from build123d import *

# Parameters (mm, degrees)
SKETCH1_W                   = 50
SKETCH1_H                   = 36
BOSS_EXTRUDE1_DEPTH         = 4
SKETCH2_W                   = 30
SKETCH2_H                   = 3
BOSS_EXTRUDE2_DEPTH         = 37
SKETCH3_R                   = 1.55
CUT_EXTRUDE1_DEPTH          = 72.867934435
SKETCH4_W                   = 16
SKETCH4_H                   = 11
CUT_EXTRUDE2_DEPTH          = 10
CUT_EXTRUDE3_DEPTH          = 10
SKETCH6_W                   = 20
SKETCH6_H                   = 12
CUT_EXTRUDE4_DEPTH          = 8
SKETCH7_W                   = 30
SKETCH7_H                   = 3
BOSS_EXTRUDE3_DEPTH         = 2
CHAMFER1_SIZE               = 2
CIRPATTERN1_COUNT           = 2
CIRPATTERN1_COPY_1_DEPTH    = 10
SKETCH9_W                   = 5
SKETCH9_H                   = 36
CUT_EXTRUDE6_DEPTH          = 10
CHAMFER2_SIZE               = 0.5
SKETCH10_W                  = 30
SKETCH10_H                  = 2
BOSS_EXTRUDE4_DEPTH         = 2
CHAMFER3_SIZE               = 2
CUT_EXTRUDE7_START          = -1.5
SKETCH12_W                  = 12.2
SKETCH12_H                  = 5.7
CUT_EXTRUDE7_DEPTH          = 7.5
CIRPATTERN2_COUNT           = 2
CIRPATTERN2_START           = -1.5
CIRPATTERN2_COPY_1_SKETCH_W = 12.2
CIRPATTERN2_COPY_1_SKETCH_H = 5.7
CIRPATTERN2_COPY_1_DEPTH    = 7.5
CHAMFER4_SIZE               = 2


with BuildPart() as part:
    # Sketch1 → Boss-Extrude1 (new body)
    with BuildSketch(Plane.XY):
        with Locations((25, 18)):
            Rectangle(SKETCH1_W, SKETCH1_H)
    extrude(amount=BOSS_EXTRUDE1_DEPTH)

    # Sketch2 → Boss-Extrude2 (add)
    with BuildSketch(Plane(origin=(0, 0, 0), x_dir=(-1, 0, 0), z_dir=(0, 0, -1))):
        with Locations((-35, 34.5)):
            Rectangle(SKETCH2_W, SKETCH2_H)
        with Locations((-35, 1.5)):
            Rectangle(SKETCH2_W, SKETCH2_H)
    extrude(amount=-BOSS_EXTRUDE2_DEPTH)

    # Sketch3 → Cut-Extrude1 (cut, through all)
    with BuildSketch(Plane(origin=(0, 36, 0), x_dir=(1, 0, 0), z_dir=(0, 1, 0))):
        with Locations(Location((40, -30, 0), (0, 0, 270))):
            Circle(SKETCH3_R)
    extrude(amount=-CUT_EXTRUDE1_DEPTH, mode=Mode.SUBTRACT)

    # Sketch4 → Cut-Extrude2 (cut)
    with BuildSketch(Plane(origin=(0, 0, 0), x_dir=(-1, 0, 0), z_dir=(0, 0, -1))):
        with Locations((-27, 18)):
            Rectangle(SKETCH4_W, SKETCH4_H)
    extrude(amount=-CUT_EXTRUDE2_DEPTH, mode=Mode.SUBTRACT)

    # Sketch5 → Cut-Extrude3 (cut)
    with BuildSketch(Plane(origin=(0, 0, 0), x_dir=(-1, 0, 0), z_dir=(0, 0, -1))):
        with BuildLine():
            Line((-44, 14.25), (-38, 14.25))
            ThreePointArc((-38, 14.25), (-36.25, 12.5), (-38, 10.75))
            Line((-38, 10.75), (-44, 10.75))
            ThreePointArc((-44, 10.75), (-45.75, 12.5), (-44, 14.25))
        make_face()
    cut_extrude3 = extrude(amount=-CUT_EXTRUDE3_DEPTH, mode=Mode.SUBTRACT)

    # Mirror1: Cut-Extrude3 across plane
    add(cut_extrude3.mirror(Plane.ZX.offset(22)), mode=Mode.SUBTRACT)

    # Sketch6 → Cut-Extrude4 (cut)
    with BuildSketch(Plane(origin=(0, 0, 0), x_dir=(-1, 0, 0), z_dir=(0, 0, -1))):
        with Locations((-52.25, 22)):
            Rectangle(SKETCH6_W, SKETCH6_H)
    cut_extrude4 = extrude(amount=-CUT_EXTRUDE4_DEPTH, mode=Mode.SUBTRACT)

    # Sketch7 → Boss-Extrude3 (add)
    with BuildSketch(Plane(origin=(0, 3, 0), x_dir=(1, 0, 0), z_dir=(0, 1, 0))):
        with Locations((35, -23.2)):
            Rectangle(SKETCH7_W, SKETCH7_H)
    boss_extrude3 = extrude(amount=BOSS_EXTRUDE3_DEPTH)

    # Mirror3: Boss-Extrude3 across plane
    add(boss_extrude3.mirror(Plane.ZX.offset(18)))

    # Chamfer1
    chamfer1_edges = [part.edges().sort_by_distance(p)[0] for p in [
        (35, 33, 21.7),
        (35, 3, 21.7),
    ]]
    chamfer(chamfer1_edges, length=CHAMFER1_SIZE - 0.0001)  # a hair under: the kernel refuses the full size

    # CirPattern1: Cut-Extrude3, Cut-Extrude4 ×2 about axis
    cirpattern1_axis = Axis((27, 18, 0), (0, 0, 1))
    add([cut_extrude3.rotate(cirpattern1_axis, i * 360 / CIRPATTERN1_COUNT) for i in range(1, CIRPATTERN1_COUNT)], mode=Mode.SUBTRACT)
    add([cut_extrude4.rotate(cirpattern1_axis, i * 360 / CIRPATTERN1_COUNT) for i in range(1, CIRPATTERN1_COUNT)], mode=Mode.SUBTRACT)

    # CirPattern1 copy 1 sketch → CirPattern1 copy 1 (cut)
    with BuildSketch(Plane(origin=(54, -8, 0), x_dir=(1, 0, 0), z_dir=(0, 0, -1))):
        with BuildLine():
            Line((-44, -14.25), (-38, -14.25))
            ThreePointArc((-38, -14.25), (-36.25, -12.5), (-38, -10.75))
            Line((-38, -10.75), (-44, -10.75))
            ThreePointArc((-44, -10.75), (-45.75, -12.5), (-44, -14.25))
        make_face()
    extrude(amount=-CIRPATTERN1_COPY_1_DEPTH, mode=Mode.SUBTRACT)

    # Sketch9 → Cut-Extrude6 (cut)
    with BuildSketch(Plane(origin=(0, 0, 0), x_dir=(-1, 0, 0), z_dir=(0, 0, -1))):
        with Locations((-2.5, 18)):
            Rectangle(SKETCH9_W, SKETCH9_H)
    extrude(amount=-CUT_EXTRUDE6_DEPTH, mode=Mode.SUBTRACT)

    # Chamfer2
    chamfer2_edges = [part.edges().sort_by_distance(p)[0] for p in [
        (41, 29.75, 0),
        (45.75, 31.5, 0),
        (36.25, 31.5, 0),
        (41, 33.25, 0),
        (50, 32, 0),
        (46.125, 28, 0),
        (46.125, 16, 0),
        (42.25, 22, 0),
        (8.25, 23.5, 0),
        (13, 25.25, 0),
        (17.75, 23.5, 0),
        (13, 21.75, 0),
        (8.25, 4.5, 0),
        (13, 2.75, 0),
        (17.75, 4.5, 0),
        (13, 6.25, 0),
        (8.375, 8, 0),
        (11.75, 14, 0),
        (8.375, 20, 0),
        (27.5, 0, 0),
        (5, 28, 0),
        (5, 4, 0),
        (27.5, 36, 0),
        (50, 8, 0),
        (35, 18, 0),
        (27, 12.5, 0),
        (19, 18, 0),
        (27, 23.5, 0),
        (45.75, 12.5, 0),
        (41, 10.75, 0),
        (36.25, 12.5, 0),
        (41, 14.25, 0),
    ]]
    chamfer(chamfer2_edges, length=CHAMFER2_SIZE)

    # Sketch10 → Boss-Extrude4 (add)
    with BuildSketch(Plane(origin=(0, 3, 0), x_dir=(1, 0, 0), z_dir=(0, 1, 0))):
        with Locations((35, -36)):
            Rectangle(SKETCH10_W, SKETCH10_H)
    boss_extrude4 = extrude(amount=BOSS_EXTRUDE4_DEPTH)

    # Mirror4: Boss-Extrude4 across plane
    add(boss_extrude4.mirror(Plane.ZX.offset(18)))

    # Chamfer3
    chamfer3_edges = [part.edges().sort_by_distance(p)[0] for p in [
        (35, 31, 37),
        (35, 5, 37),
    ]]
    chamfer(chamfer3_edges, length=CHAMFER3_SIZE - 0.0001)  # a hair under: the kernel refuses the full size

    # Sketch12 → Cut-Extrude7 (cut)
    with BuildSketch(Plane.XY.offset(4).offset(CUT_EXTRUDE7_START)):
        with Locations((13, 23.5)):
            Rectangle(SKETCH12_W, SKETCH12_H)
    cut_extrude7 = extrude(amount=CUT_EXTRUDE7_DEPTH, mode=Mode.SUBTRACT)

    # Mirror5: Cut-Extrude7 across plane
    add(cut_extrude7.mirror(Plane(origin=(0, 14, 0), x_dir=(0, 0, 1), z_dir=(0, -1, 0))), mode=Mode.SUBTRACT)

    # CirPattern2: Cut-Extrude7 ×2 about axis
    cirpattern2_axis = Axis((27, 18, 0), (0, 0, 1))
    for i in range(1, CIRPATTERN2_COUNT):
        add(cut_extrude7.rotate(cirpattern2_axis, i * 360 / CIRPATTERN2_COUNT), mode=Mode.SUBTRACT)

    # CirPattern2 copy 1 sketch → CirPattern2 copy 1 (cut)
    with BuildSketch(Plane(origin=(54, 8, 4), x_dir=(-1, 0, 0), z_dir=(0, 0, 1)).offset(CIRPATTERN2_START)):
        with Locations((13, -23.5)):
            Rectangle(CIRPATTERN2_COPY_1_SKETCH_W, CIRPATTERN2_COPY_1_SKETCH_H)
    extrude(amount=CIRPATTERN2_COPY_1_DEPTH, mode=Mode.SUBTRACT)

    # Chamfer4
    chamfer4_edges = [part.edges().sort_by_distance(p)[0] for p in [
        (48.55, 33, 4),
        (35, 3, 4),
        (27.45, 33, 4),
    ]]
    chamfer(chamfer4_edges, length=CHAMFER4_SIZE)


solid = part.part
Here's how the part is built. I have some questions about the finished solid (model axes, mm). A direction names the side the tool comes from. Round coordinates to 2 decimals unless told otherwise and drop trailing zeros. Loops run counter-clockwise (first coordinate to the right, second up) from the corner with the lowest first, then second, coordinate; pieces in that order, holes last.
1. We'd pull the mould along X, two halves only. Please class faces 1 (the face through (19, 18, 2)), 2 (the face through (27, 26, 0)), 3 (the face through (20, 2, 21)): +X half, -X half, draft (parallel to the pull), parting line (faces both ways), or undercut.
Answer list:
face 1: undercut
face 2: draft
face 3: -X half
2. For P1, Ø1.5, axis at x = 33, y = 13, coming from the +Z side; P2, Ø1, axis at x = 29.5, y = 4, coming from the +Z side, each with a flat end and sliding along its axis, tell me the tip position at first contact or that it passes through.
Answer list:
P1: stops at z = 4
P2: stops at z = 36.5
3. If I drill on line 1 along X through (y, z) = (34, 30); line 2 along Y through (x, z) = (42.5, 17); line 3 along Y through (x, z) = (28, 24), over which ranges is the centre line in solid material (lowest first)?
Answer list:
line 1: x = 20 to 38.45, 41.55 to 50
line 2: y = 0 to 3, 33 to 36
line 3: y = 0 to 5, 31 to 36
4. If we section it at D-D on x = 40: Count the separate pieces of the cut face and the enclosed holes in it, plus the area to 3 significant figures.
Answer list:
separate pieces: 5
enclosed holes: 0
area: 302 mm2
5. Which directions (+Z, -Z, +X, -X, +Y, -Y) give clear straight access to the entire face, cutting with the end or side of a thin tool? Please do faces 4 (the face through (13, 7.35, 3)), 5 (the face through (41.09, 29.56, 2.5)), 6 (the face through (17.885, 4.541, 0.365)), 7 (the face through (35, 4, 36)).
Answer list:
face 4: +Z
face 5: none
face 6: -Z
face 7: +Z, +X, -X
6. If we section it at B-B on y = 18: Write out the boundary of the cut face in (x, z).
Answer list:
outline: (11.75, 0.5) - (12.25, 0) - (18.5, 0) - (19, 0.5) - (19, 4) - (11.75, 4) - close; (35, 0.5) - (35.5, 0) - (41.75, 0) - (42.25, 0.5) - (42.25, 4) - (35, 4) - close
7. If we section it at A-A on z = 30: Write out the boundary of the cut face in (x, y).
Answer list:
outline: (20, 0) - (38.45, 0) - (38.45, 3) - (20, 3) - close; (20, 33) - (38.45, 33) - (38.45, 36) - (20, 36) - close; (41.55, 0) - (50, 0) - (50, 3) - (41.55, 3) - close; (41.55, 33) - (50, 33) - (50, 36) - (41.55, 36) - close
8. If we section it at C-C on z = 15.5: Write out the boundary of the cut face in (x, y), plus the area to 3 significant figures.
Answer list:
outline: (20, 0) - (50, 0) - (50, 3) - (20, 3) - close; (20, 33) - (50, 33) - (50, 36) - (20, 36) - close
area: 180 mm2
